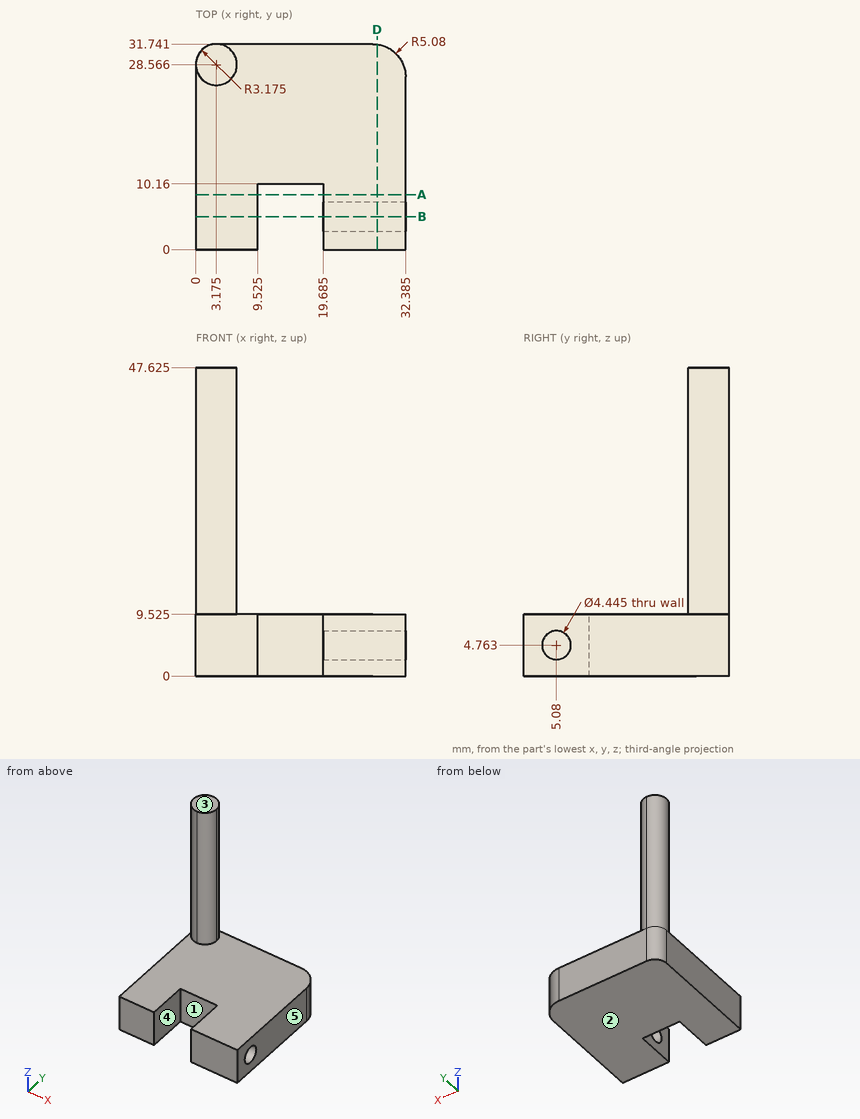
Geometry: see drawing. Coordinates: mm, zero at the bounding-box minimum. A direction names the side the tool comes from. Give positions to 0.01 mm unless a question says otherwise; leave off trailing zeros. Order: outer loops, then holes, each group sorted by start corner. A loop starts at its lowest first (then second) coordinate and runs counter-clockwise, first axis right, second up.
Q1. Section A-A on y = 8.5. Output: boundary loops of the cut face in (x, z) (1 decimal), and give its area (3 significant figures).
Checked values:
outline: (0, 0) - (9.5, 0) - (9.5, 9.5) - (0, 9.5) - close; (19.7, 0) - (32.4, 0) - (32.4, 9.5) - (19.7, 9.5) - close
area: 212 mm2
Q2. Contact query for flat-ended pins moving along their axis: pin 1 Ø6 at (y, z) = (13, 5) entering from -X; pin 2 Ø16 at (x, y) = (13, 16) entering from +Z (1 decimal); pin 3 Ø6 at (x, z) = (12, 23.5) entering from -Y. Output: stop coordinate, or through.
Checked values:
pin 1: stops at x = 0
pin 2: stops at z = 9.5
pin 3: passes through
Q3. Ray query, probe 1 along Z at (x, y) = (28, 5) (1 decimal); probe 2 along Z at (x, y) = (20.5, 10) (1 decimal); probe 3 along Y at (x, z) = (3, 22) (1 decimal). Return the intervals inside material, ascending.
Checked values:
probe 1: z = 0 to 2.5, 7 to 9.5
probe 2: z = 0 to 9.5
probe 3: y = 25.4 to 31.7
Q4. Section B-B on y = 5.08. Output: boundary loops of the cut face in (x, z) (1 decimal).
Checked values:
outline: (0, 0) - (9.5, 0) - (9.5, 9.5) - (0, 9.5) - close; (19.7, 0) - (32.4, 0) - (32.4, 2.5) - (19.7, 2.5) - close; (19.7, 7) - (32.4, 7) - (32.4, 9.5) - (19.7, 9.5) - close
Q5. Set-up query: the marked faces 1 and 2. Return all of +Z, -Z, +X, -X, +Y, -Y with unobstructed straight access to the full face (end or side cutting, diameter ignored); none if empty.
Checked values:
face 1: +Z, -Z, -Y
face 2: -Z, +X, -X, +Y, -Y
Q6. Section D-D on x = 28. Output: boundary loops of the cut face in (y, z) (1 decimal).
Checked values:
outline: (0, 0) - (31.7, 0) - (31.7, 9.5) - (0, 9.5) - close; hole circle Ø4.4 at (5.1, 4.8)
Q7. Draft query along X for the marked faces 3, 4 and 5. Return one class per face: +X half, -X half, draft (parallel to the pull), parting line (faces both ways), or undercut.
Checked values:
face 3: draft
face 4: undercut
face 5: +X half
